Source: CAD feature listing. Evaluate the final solid. Frame: model axes, mm. Face numbers are marked on the shaded views. A direction names the side the tool comes from. Round coordinates to 2 decimals unless told otherwise and drop trailing zeros. Order: outer loops, then holes, each group sorted by start corner. A loop starts at its lowest first (then second) coordinate and runs counter-clockwise, first axis right, second up. Notation, with made-up numbers: M -16,45.5 L 9,45.5 A34 ccw 9,84.5 Z; hole C 58,3.25 d2. An arc over 180 degrees is marked long. Answer in a Markdown table with one row per item. Add a question column.
```python
from build123d import *

# Parameters (mm, degrees)
F0_R     = 12.7
F1_DEPTH = 25.4
F2_R     = 12.7
F3_DEPTH = 25.4
F4_R     = 12.7


with BuildPart() as f1:
    # F0 (on Front) → F1 (new body)
    with BuildSketch(Plane.XZ):
        with BuildLine():
            Line((50.6083145556, -19.7611999094), (-36.7538123162, 39.3731284323))
            ThreePointArc((-36.7538123162, 39.3731284323), (-62.897944776, 40.7753994034), (-76.3916854444, 18.3388000906))
            Line((-76.3916854444, 18.3388000906), (-76.3916854444, -32.4611999094))
            Line((-76.3916854444, -32.4611999094), (50.6083145556, -32.4611999094))
            Line((50.6083145556, -32.4611999094), (50.6083145556, -19.7611999094))
        make_face()
        with Locations((-50.9916854444, 18.3388000906)):
            Circle(F0_R, mode=Mode.SUBTRACT)
    extrude(amount=F1_DEPTH)

    # F2 (on face) → F3 (join)
    with BuildSketch(Plane.XZ.offset(25.4)):
        with BuildLine():
            Line((-25.5916854444, -19.7611999094), (-25.5916854444, 18.3388000906))
            ThreePointArc((-25.5916854444, 18.3388000906), (-50.9916854444, 43.7388000906), (-76.3916854444, 18.3388000906))
            Line((-76.3916854444, 18.3388000906), (-76.3916854444, -19.7611999094))
            Line((-76.3916854444, -19.7611999094), (-76.3916854444, -32.4611999094))
            Line((-76.3916854444, -32.4611999094), (50.6083145556, -32.4611999094))
            Line((50.6083145556, -32.4611999094), (50.6083145556, -19.7611999094))
            Line((50.6083145556, -19.7611999094), (-25.5916854444, -19.7611999094))
        make_face()
        with Locations((-50.9916854444, 18.3388000906)):
            Circle(F2_R, mode=Mode.SUBTRACT)
    extrude(amount=F3_DEPTH)

    # F4
    f4_edges = [f1.edges().sort_by_distance(p)[0] for p in [
        (50.608315, -50.8, -26.1112),
    ]]
    fillet(f4_edges, radius=F4_R)


solid = f1.part
```
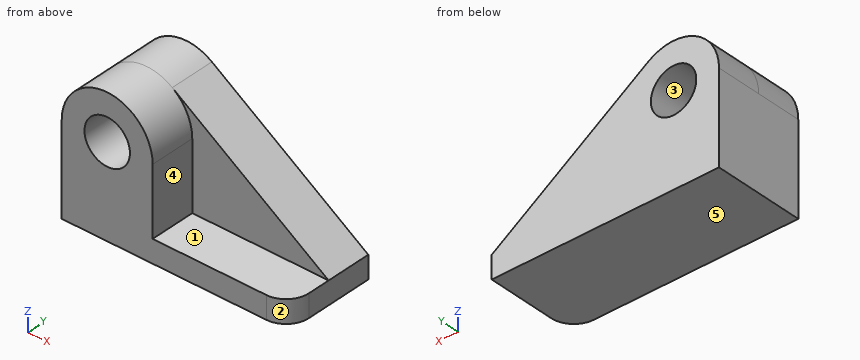
(1) Cut plane B-B (z = 10.5). Return loops of the section in (x, y), and give its area (3 significant figures).
(2) Cut plane D-D (y = -10). Return loops of the section in (x, z), and give its area (3 significant figures).
(3) Line query: line 1 (Y direction, x = 33, z = -11.5); line 2 (X direction, y = -25, z = 10); line 3 (Z direction, x = -57.5, y = -6.5). Output: solid intervals per line, ascending. Write a range as from..to.
(4) Cut plane C-C (x = -69). Return loops of the section in (y, z), and give its area (3 significant figures).
(5) Cut plane A-A (y = -44). Return loops of the section in (x, z).
(6) Pin query (flat end, axial travel): pin 1 (4 mm diameter, centred on x = -4.5, z = -4, fed in from -Y); pin 2 (6 mm diameter, centred on x = 17.5, y = -40.5, fed in from +Z); pin 3 (2 mm diameter, centred on x = -45.5, y = -23.5, fed in from +Z); pin 4 (10 mm diameter, centred on x = 3.5, z = 22.5, fed in from -Y). Return the tip coordinate at first contact, or that it passes through.
(7) Access query for the marked faces 4 and 5. Directions: +Z, -Z, +X, -X, +Y, -Y. A direction counts if a zero-diameter tool reaches every point of the face in a straight line with its end or side. Return the directions, or none.
(8) Draft query along Z for the marked faces 1, 2 and 3. Return one class per face: +Z half, -Z half, draft (parallel to the pull), parting line (faces both ways), or undercut.
Answer list:
| question | item | result |
|---|---|---|
| 1 | outline | M -76.39,-50.8 L -60.98,-50.8 L -60.98,0 L -76.39,0 Z; M -41,-50.8 L -25.59,-50.8 L -25.59,-25.4 L 5.9,-25.4 L 5.9,0 L -41,0 Z |
| 1 | area | 2,370 mm² |
| 2 | outline | M -76.39,-32.46 L 50.61,-32.46 L 50.61,-19.76 L -36.75,39.37 A25.4 ccw -76.39,18.34 Z; hole C -50.99,18.34 d25.4 |
| 2 | area | 6,050 mm² |
| 3 | line 1 | -25.4..0 |
| 3 | line 2 | -76.39..-60.57, -41.41..6.64 |
| 3 | line 3 | -32.46..7.43, 29.24..42.89 |
| 4 | outline | M -50.8,-32.46 L 0,-32.46 L 0,36.25 L -50.8,36.25 Z |
| 4 | area | 3,490 mm² |
| 5 | outline | M -76.39,-32.46 L 49.15,-32.46 L 49.15,-19.76 L -25.59,-19.76 L -25.59,18.34 A25.4 ccw -76.39,18.34 Z; hole C -50.99,18.34 d25.4 |
| 6 | pin 1 | y = -25.4 |
| 6 | pin 2 | z = -19.76 |
| 6 | pin 3 | z = 43.34 |
| 6 | pin 4 | through |
| 7 | face 4 | +Z, +X, -Y |
| 7 | face 5 | -Z, +X, -X, +Y, -Y |
| 8 | face 1 | +Z half |
| 8 | face 2 | draft |
| 8 | face 3 | undercut |
